from build123d import *

# Parameters (mm, degrees)
F0_R     = 68.5822054127
F1_DEPTH = 148.59
F2_T     = -2.54


# Not quite as in the source:
# - a fillet or chamfer that OpenCascade refuses, or shapes differently, is made with other operations: its cross-section is extruded or revolved along the edge and cut away or added


with BuildPart() as f1:
    # F0 (on Top) → F1 (new body)
    with BuildSketch(Plane.XY):
        Circle(F0_R)
    extrude(amount=-F1_DEPTH)

    # F2
    f2_openings = [f1.faces().sort_by_distance(p)[0] for p in [
        (0, 0, 0),
    ]]
    offset(amount=F2_T, openings=f2_openings)

    # F3: fillet of radius 31.273722487 on 1 edges, made by hand

    # F3_s1 → F3_t2 (revolve, cut)
    with BuildSketch(Plane.XZ):
        with BuildLine():
            ThreePointArc((68.5822054127, -12.34580537), (67.9406243892, -6.0436130881), (66.0422054127, 0))
            Line((66.0422054127, 0), (66.6168798625, 0.2469161074))
            ThreePointArc((66.6168798625, 0.2469161074), (67.3122054127, 0.6254744497), (68.5822054127, 0.6254744497))
            Line((68.5822054127, 0.6254744497), (69.2076798625, 0))
            Line((69.2076798625, 0), (69.2076798625, -12.34580537))
            Line((69.2076798625, -12.34580537), (68.5822054127, -12.34580537))
        make_face()
    revolve(axis=Axis((0, 0, 0), (0, 0, 1)), mode=Mode.SUBTRACT)


solid = f1.part
Check sheet for the modelled part. Datum: model origin and axes. Units: mm. Give positions to 0.01 mm unless a question says otherwise; leave off trailing zeros. Write each loop counter-clockwise with the first axis right and the second up, starting at its lowest first coordinate (ties: lowest second). Pieces come first, ordered by that corner, then holes. Notation, with made-up numbers: (47, 5) -> (64, 5) arc R7 ccw to (64, 17) -> close; hole circle Ø3 at (15, 14.5). An arc over 180 degrees is marked (long way). Write item = value, one per line.
Item 1: Release check for a two-part mould opening along X. For faces 1 (the cylindrical face through (36.87, 57.83, -79.51)), 2 (the flat face through (-1, 1, -148.59)), 3 (the cylindrical face through (62.99, 19.84, -72)) record: +X half, -X half, draft (parallel to the pull), parting line (faces both ways), or undercut.
Output:
face_1 = parting line
face_2 = draft
face_3 = undercut
Item 2: Scan lines: probe 1 along Y at (x, z) = (0, -45); probe 2 along Z at (x, y) = (-36, 14); probe 3 along X at (y, z) = (5.5, -115.5). Record each from-to range of solid material in increasing order. Write a range as from..to.
Output:
probe_1 = -68.58..-66.04, 66.04..68.58
probe_2 = -148.59..-146.05
probe_3 = -68.36..-65.81, 65.81..68.36
Item 3: Sectioned sample at B-B on z = -59. Record the boundary of the cut face in (x, y), and give its area (3 significant figures).
Output:
outline = circle Ø137.16 at (0, 0); hole circle Ø132.08 at (0, 0)
area = 1,070 mm^2
Item 4: Gauge pin test, flat ends, axial feed: pin 1 (10 mm diameter, centred on y = 17.5, z = -88.5, fed in from -X); pin 2 (4 mm diameter, centred on y = 48.5, z = -114, fed in from +X); pin 3 (12 mm diameter, centred on y = -24, z = -59.5, fed in from +X). Record the tip position at first contact, or that the pin passes through.
Output:
pin_1 = -67.43
pin_2 = 50.41
pin_3 = 66.18
Item 5: Sectioned sample at A-A on x = 0. Record the boundary of the cut face in (y, z), and give its area (3 significant figures).
Output:
outline = (-68.58, -148.59) -> (68.58, -148.59) -> (68.58, -12.35) arc R31.27 ccw to (66.04, 0) -> (66.04, -146.05) -> (-66.04, -146.05) -> (-66.04, 0) arc R31.27 ccw to (-68.58, -12.35) -> close
area = 1,070 mm^2
